```python
from build123d import *

# Parameters (mm, degrees)
SKETCH3_W = 1.2
SKETCH3_H = 6.2


with BuildPart() as part:
    # Sweep1: sweep along a path in Sketch2
    with BuildLine(Plane.XY) as sweep1_path:
        Line((-6.448403422, -0.111551706), (-11.600882618, 297.734761881))
        ThreePointArc((-11.600882618, 297.734761881), (-13.342957561, 301.819476981), (-17.439980035, 303.532407044))
        Line((-17.439980035, 303.532407044), (-209.956343171, 305.490953375))
        ThreePointArc((-209.956343171, 305.490953375), (-217.025815722, 312.63271234), (-209.956343171, 319.774471304))
        Line((-209.956343171, 319.774471304), (-17.439980035, 321.733017635))
        ThreePointArc((-17.439980035, 321.733017635), (-13.374840603, 323.414530272), (-11.603110065, 327.441168355))
        Line((-11.603110065, 327.441168355), (-6.445968569, 486.209379269))
        ThreePointArc((-6.445968569, 486.209379269), (0.101636768, 492.448567317), (6.449365306, 486.006134116))
        Line((6.449365306, 486.006134116), (6.600002669, 327.627100738))
        ThreePointArc((6.600002669, 327.627100738), (8.294727162, 323.494393797), (12.399704541, 321.733564874))
        Line((12.399704541, 321.733564874), (200.716608272, 318.531859805))
        ThreePointArc((200.716608272, 318.531859805), (206.516312813, 312.63271234), (200.716608272, 306.733564874))
        Line((200.716608272, 306.733564874), (12.399704541, 303.531859805))
        ThreePointArc((12.399704541, 303.531859805), (8.293806439, 301.770095054), (6.600000756, 297.635698295))
        Line((6.600000756, 297.635698295), (6.449367397, -0.003263988))
        ThreePointArc((6.449367397, -0.003263988), (0.054146005, -6.449140926), (-6.448403422, -0.111551706))
    # Sketch3 → Sweep1 (sweep)
    with BuildSketch(Plane(origin=(0, 0, 0), x_dir=(1, 0, 0), z_dir=(0, 1, 0))):
        with Locations((7.049367397, 3.1)):
            Rectangle(SKETCH3_W, SKETCH3_H)
    sweep(path=sweep1_path.line)


solid = part.part
```
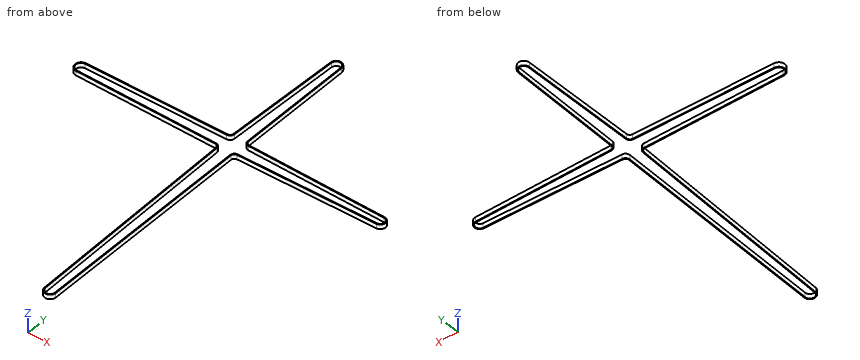
For this review, take the finished solid that the model builds, in its own axes (mm). Give positions to 0.01 mm unless a question says otherwise; leave off trailing zeros. Write each loop counter-clockwise with the first axis right and the second up, starting at its lowest first coordinate (ties: lowest second). Pieces come first, ordered by that corner, then holes. Notation, with made-up numbers: M 21.5,-40 L 53.5,-40 A33 ccw 53.5,-8 Z; hole C -32,27.25 d11. An arc over 180 degrees is marked long. Answer as a JSON object with one key per item and string values. Group by question number.
Item 1: For probe 1 along Y at (x, z) = (13.5, -2.5); probe 2 along Y at (x, z) = (131, -3.5); probe 3 along X at (y, z) = (17, -1), list the stretches that pass through material, from the lowest coordinate up. Write a range as [from, to].
Item 2: Consider section C-C on y = 266. Write out the cut boundary in (x, z), plus the area to 3 significant figures.
Item 3: For pin 1 Ø1.5 at (x, z) = (145.5, -4.5) entering from +Y; pin 2 Ø10 at (x, y) = (122, 296.5) entering from +Z; pin 3 Ø10 at (x, y) = (67, 307.5) entering from -Z; pin 4 Ø1.5 at (y, z) = (400, -3.5) entering from -X, all flat-tipped, find the tip position at first contact; note any pin that passes through.
Item 4: Consider section A-A on x = 0. Write out the cut boundary in (y, z), plus the area to 3 significant figures.
Check result:
{
 "1": {"probe 1": "y = [302.35, 303.55], [321.71, 322.92]", "probe 2": "y = [304.35, 305.55], [319.72, 320.92]", "probe 3": "x = [-7.94, -6.74], [6.46, 7.66]"},
 "2": {"outline": "M -12.25,-6.2 L -11.05,-6.2 L -11.05,0 L -12.25,0 Z; M 6.58,-6.2 L 7.78,-6.2 L 7.78,0 L 6.58,0 Z", "area": "14.9 mm^2"},
 "3": {"pin 1": "stops at y = 320.68", "pin 2": "passes through", "pin 3": "stops at z = -6.2", "pin 4": "stops at x = -10.47"},
 "4": {"outline": "M -7.65,-6.2 L -6.45,-6.2 L -6.45,0 L -7.65,0 Z; M 492.45,-6.2 L 493.65,-6.2 L 493.65,0 L 492.45,0 Z", "area": "14.9 mm^2"}
}
